```python
from build123d import *

# Parameters (mm, degrees)
F0_W     = 58
F0_H     = 46
F1_DEPTH = 1.5
F2_W     = 11
F2_H     = 7
F3_DEPTH = 1.501
F4_W     = 13
F4_H     = 9
F4_W_2   = 11
F4_H_2   = 7
F5_DEPTH = 1.501
F0_W_2   = 62
F0_H_2   = 50
F6_DEPTH = 3


with BuildPart() as f1:
    # F0 (on Top) → F1 (new body)
    with BuildSketch(Plane.XY):
        Rectangle(F0_W, F0_H)
    extrude(amount=F1_DEPTH)

    # F2 (on face) → F3 (cut, through all)
    with BuildSketch(Plane.XY.offset(1.5)):
        with Locations((-21, 16.5)):
            Rectangle(F2_W, F2_H)
        with Locations((-7, 16.5)):
            Rectangle(F2_W, F2_H)
        with Locations((7, 16.5)):
            Rectangle(F2_W, F2_H)
        with Locations((21, 16.5)):
            Rectangle(F2_W, F2_H)
        with Locations((-20.923837, 5.500264)):
            Rectangle(F2_W, F2_H)
        with Locations((-6.923837, 5.500264)):
            Rectangle(F2_W, F2_H)
        with Locations((7.076163, 5.500264)):
            Rectangle(F2_W, F2_H)
        with Locations((21.076163, 5.500264)):
            Rectangle(F2_W, F2_H)
        with Locations((-20.847673, -5.499473)):
            Rectangle(F2_W, F2_H)
        with Locations((-6.847673, -5.499473)):
            Rectangle(F2_W, F2_H)
        with Locations((7.152327, -5.499473)):
            Rectangle(F2_W, F2_H)
        with Locations((21.152327, -5.499473)):
            Rectangle(F2_W, F2_H)
        with Locations((-20.77151, -16.499209)):
            Rectangle(F2_W, F2_H)
        with Locations((-6.77151, -16.499209)):
            Rectangle(F2_W, F2_H)
        with Locations((7.22849, -16.499209)):
            Rectangle(F2_W, F2_H)
        with Locations((21.22849, -16.499209)):
            Rectangle(F2_W, F2_H)
    extrude(amount=-F3_DEPTH, mode=Mode.SUBTRACT)

    # F4 (on face) → F5 (cut, through all)
    with BuildSketch(Plane.XY.offset(1.5)):
        with Locations((-21, 16.5)):
            Rectangle(F4_W, F4_H)
        with Locations((-21, 16.5)):
            Rectangle(F4_W_2, F4_H_2, mode=Mode.SUBTRACT)
        with Locations((-7, 16.5)):
            Rectangle(F4_W, F4_H)
        with Locations((-7, 16.5)):
            Rectangle(F4_W_2, F4_H_2, mode=Mode.SUBTRACT)
        with Locations((7, 16.5)):
            Rectangle(F4_W, F4_H)
        with Locations((7, 16.5)):
            Rectangle(F4_W_2, F4_H_2, mode=Mode.SUBTRACT)
        with Locations((21, 16.5)):
            Rectangle(F4_W, F4_H)
        with Locations((21, 16.5)):
            Rectangle(F4_W_2, F4_H_2, mode=Mode.SUBTRACT)
        with Locations((-21, 5.5)):
            Rectangle(F4_W, F4_H)
        with Locations((-20.923837, 5.500264)):
            Rectangle(F4_W_2, F4_H_2, mode=Mode.SUBTRACT)
        with Locations((7, 5.5)):
            Rectangle(F4_W, F4_H)
        with Locations((7.076163, 5.500264)):
            Rectangle(F4_W_2, F4_H_2, mode=Mode.SUBTRACT)
        with Locations((-7, 5.5)):
            Rectangle(F4_W, F4_H)
        with Locations((-6.923837, 5.500264)):
            Rectangle(F4_W_2, F4_H_2, mode=Mode.SUBTRACT)
        with Locations((21, 5.5)):
            Rectangle(F4_W, F4_H)
        with Locations((21.076163, 5.500264)):
            Rectangle(F4_W_2, F4_H_2, mode=Mode.SUBTRACT)
        with Locations((-21, -5.5)):
            Rectangle(F4_W, F4_H)
        with Locations((-20.847673, -5.499473)):
            Rectangle(F4_W_2, F4_H_2, mode=Mode.SUBTRACT)
        with Locations((-7, -5.5)):
            Rectangle(F4_W, F4_H)
        with Locations((-6.847673, -5.499473)):
            Rectangle(F4_W_2, F4_H_2, mode=Mode.SUBTRACT)
        with Locations((7, -5.5)):
            Rectangle(F4_W, F4_H)
        with Locations((7.152327, -5.499473)):
            Rectangle(F4_W_2, F4_H_2, mode=Mode.SUBTRACT)
        with Locations((21, -5.5)):
            Rectangle(F4_W, F4_H)
        with Locations((21.152327, -5.499473)):
            Rectangle(F4_W_2, F4_H_2, mode=Mode.SUBTRACT)
        with Locations((-21, -16.5)):
            Rectangle(F4_W, F4_H)
        with Locations((-20.77151, -16.499209)):
            Rectangle(F4_W_2, F4_H_2, mode=Mode.SUBTRACT)
        with Locations((-7, -16.5)):
            Rectangle(F4_W, F4_H)
        with Locations((-6.77151, -16.499209)):
            Rectangle(F4_W_2, F4_H_2, mode=Mode.SUBTRACT)
        with Locations((7, -16.5)):
            Rectangle(F4_W, F4_H)
        with Locations((7.22849, -16.499209)):
            Rectangle(F4_W_2, F4_H_2, mode=Mode.SUBTRACT)
        with Locations((21, -16.5)):
            Rectangle(F4_W, F4_H)
        with Locations((21.22849, -16.499209)):
            Rectangle(F4_W_2, F4_H_2, mode=Mode.SUBTRACT)
    extrude(amount=-F5_DEPTH, mode=Mode.SUBTRACT)

    # F0 (on Top) → F6 (join)
    with BuildSketch(Plane.XY):
        Rectangle(F0_W_2, F0_H_2)
        Rectangle(F0_W, F0_H, mode=Mode.SUBTRACT)
    extrude(amount=F6_DEPTH)


solid = f1.part
```
Input: part model. Units: mm. Frame: model coordinates. A direction names the side the tool comes from. Coordinates: 2 decimals unless noted, no trailing zeros. Loops run counter-clockwise (first coordinate to the right, second up) from the corner with the lowest first, then second, coordinate; pieces in that order, holes last. Notation, with made-up numbers: M 22,57.25 L 58,57.25 A33 ccw 58,90.25 Z; hole C 12,-22 d4. An arc over 180 degrees is marked long. Use a Markdown table: item, result. Add a question column.
1) Section C-C, the plane y = -8. Return the cut outline in (x, z), plus the area to 3 significant figures.
2) Section B-B, the plane z = 2.35. Return the cut outline in (x, y), plus the area to 3 significant figures.
3) Draft query along Y for faces 3 (the flat face through (-13.5, 5, 1)), 4 (the flat face through (-2, -24, 3)). Return one class per face: +Y half, -Y half, draft (parallel to the pull), parting line (faces both ways), or undercut.
4) Line query: L1, parallel to X at y = 1.5, z = 0.25; L2, parallel to Y at x = 8.5, z = 0.85; L3, parallel to X at y = -14.5, z = 2.2. Output: solid intervals per line, ascending. Write a range as from..to.
5) Set-up query: faces 1 (the flat face through (29, 0, 2)), 2 (the flat face through (0.5, -17, 1)). Return all of +Z, -Z, +X, -X, +Y, -Y with unobstructed straight access to the full face (end or side cutting, diameter ignored); none if empty.
6) Section A-A, the plane x = -24.5. Return the cut outline in (y, z), plus the area to 3 significant figures.
7) Pin query (flat end, axial travel): P1, Ø4, axis at x = 11, y = 13.5, coming from the +Z side; P2, Ø1.5, axis at x = -14, y = 14.5, coming from the -Z side. Return the tip coordinate at first contact, or that it passes through.
Answer below:
| question | item | result |
|---|---|---|
| 1 | outline | M -31,0 L -27.5,0 L -27.5,1.5 L -29,1.5 L -29,3 L -31,3 Z; M -14.5,0 L -13.5,0 L -13.5,1.5 L -14.5,1.5 Z; M -0.5,0 L 0.5,0 L 0.5,1.5 L -0.5,1.5 Z; M 13.5,0 L 14.5,0 L 14.5,1.5 L 13.5,1.5 Z; M 27.5,0 L 31,0 L 31,3 L 29,3 L 29,1.5 L 27.5,1.5 Z |
| 1 | area | 21.0 mm2 |
| 2 | outline | M -31,-25 L 31,-25 L 31,25 L -31,25 Z; hole M -29,-23 L 29,-23 L 29,23 L -29,23 Z |
| 2 | area | 432 mm2 |
| 3 | face 3 | undercut |
| 3 | face 4 | draft |
| 4 | L1 | -31..-27.5, -14.5..-13.5, -0.5..0.5, 13.5..14.5, 27.5..31 |
| 4 | L2 | -25..-21, -12..-10, -1..1, 10..12, 21..25 |
| 4 | L3 | -31..-29, 29..31 |
| 5 | face 1 | +Z |
| 5 | face 2 | +Z, -Z |
| 6 | outline | M -25,0 L -21,0 L -21,1.5 L -23,1.5 L -23,3 L -25,3 Z; M -12,0 L -10,0 L -10,1.5 L -12,1.5 Z; M -1,0 L 1,0 L 1,1.5 L -1,1.5 Z; M 10,0 L 12,0 L 12,1.5 L 10,1.5 Z; M 21,0 L 25,0 L 25,3 L 23,3 L 23,1.5 L 21,1.5 Z |
| 6 | area | 27.0 mm2 |
| 7 | P1 | z = 1.5 |
| 7 | P2 | z = 0 |
